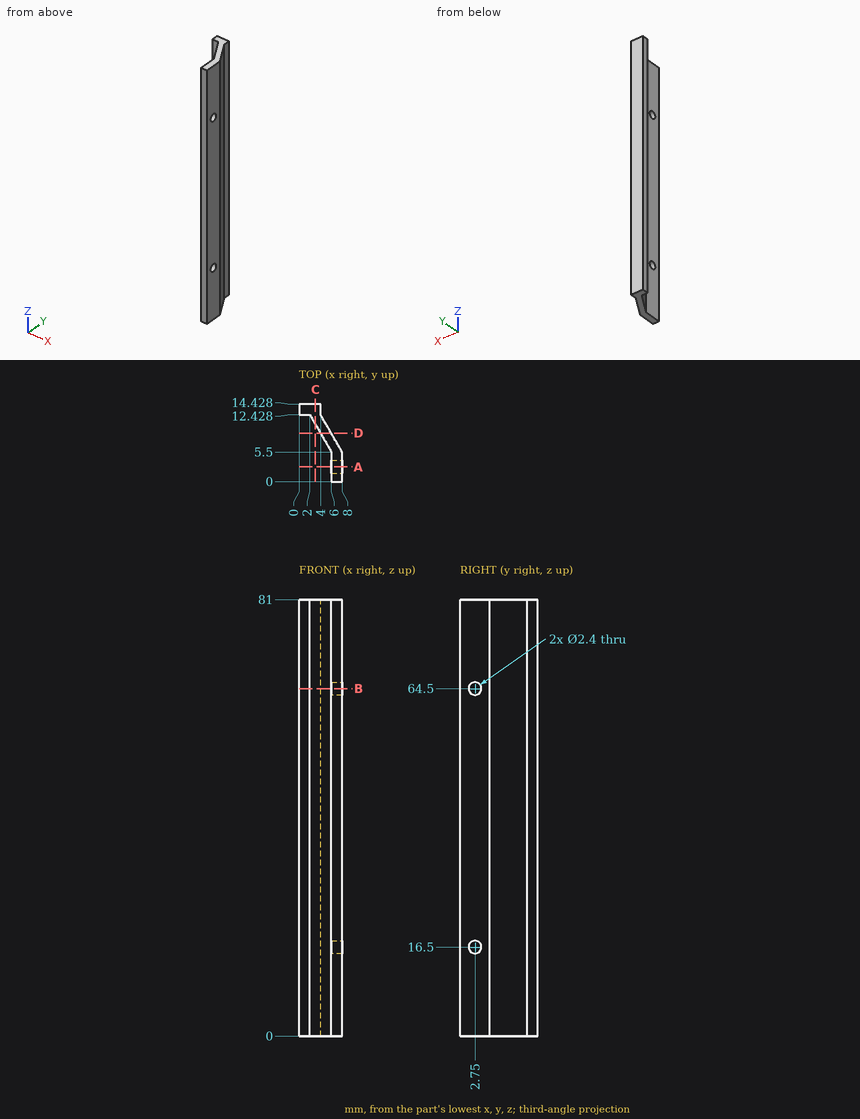
Input: dimensioned drawing with shaded views. Units: mm. Origin: part minimum x, y, z. Give positions to 0.01 mm unless a question says otherwise; leave off trailing zeros. Order: outer loops, then holes, each group sorted by start corner. A loop starts at its lowest first (then second) coordinate and runs counter-clockwise, first axis right, second up.
(1) Section query C-C (x = 3). Return the cut outline in (y, z), plus the area to 3 significant figures.
(2) Section query A-A (y = 2.75). Return the cut outline in (x, z).
(3) Contact query for flat-ended pins moving along their axis: P1, Ø0.6, axis at x = 1, z = 50.5, coming from the -Y side; P2, Ø1.6, axis at y = 13.5, z = 46.5, coming from the +X side; P3, Ø1.6, axis at y = 3, z = 29, coming from the -X side. Output: stop coordinate, or through.
(4) Material intervals for line 1 along X through (y, z) = (13.5, 73); line 2 along Y through (x, z) = (1, 24); line 3 along X through (y, z) = (4.5, 18), sorted ascending.
(5) Section query D-D (y = 9). Return the cut outline in (x, z).
(6) Section query B-B (z = 64.5). Return the cut outline in (x, y).
Outcome:
1. outline: (10.7, 0) - (14.43, 0) - (14.43, 81) - (10.7, 81) - close
1. area: 302 mm2
2. outline: (6, 0) - (8, 0) - (8, 15.3) - (6, 15.3) - close; (6, 17.7) - (8, 17.7) - (8, 63.3) - (6, 63.3) - close; (6, 65.7) - (8, 65.7) - (8, 81) - (6, 81) - close
3. P1: stops at y = 12.43
3. P2: stops at x = 4
3. P3: stops at x = 6
4. line 1: x = 0 to 4
4. line 2: y = 12.43 to 14.43
4. line 3: x = 6 to 8
5. outline: (3.98, 0) - (5.98, 0) - (5.98, 81) - (3.98, 81) - close
6. outline: (0, 12.43) - (2, 12.43) - (6, 5.5) - (6, 3.95) - (8, 3.95) - (8, 5.5) - (4, 12.43) - (4, 14.43) - (0, 14.43) - close; (6, 0) - (8, 0) - (8, 1.55) - (6, 1.55) - close
